Autodesk Inventor part; units mm, degrees
ref_plane "YZ Plane" through (0, 0, 0) normal (1, 0, 0) x (0, 1, 0)
ref_plane "XZ Plane" through (0, 0, 0) normal (0, 1, 0) x (-1, 0, 0)
ref_plane "XY Plane" through (0, 0, 0) normal (0, 0, 1) x (1, 0, 0)
sketch "Эскиз1" plane through (0, 0, 0) normal (0, 0, 1) x (1, 0, 0)
  line L0 (0, 0) -> (34.5, 0)
  line L1 (34.5, 0) -> (34.5, 9.5)
  line L2 (34.5, 9.5) -> (0, 9.5)
  line L3 (0, 9.5) -> (0, 0)
  line L4 (3, 9.5) -> (3, 0)
  line L5 (31.5, 9.5) -> (31.5, 0)
  line L6 (3, 3) -> (31.5, 3)
  dimension "d0" = 34.5
  dimension "d1" = 9.5
  dimension "d2" = 3
  dimension "d3" = 3
  dimension "d4" = 3
extrude "Выдавливание1" add sketch "Эскиз1" along normal blind 388 contours L3 L2 L4 L0 | L4 L6 L5 L0 | L5 L2 L1 L0
sketch "Эскиз2" plane through (0, 0, 0) normal (0, -1, 0) x (1, 0, 0)
  line L0 (0, 0) -> (34.5, 0)
  line L1 (34.5, 0) -> (34.5, 388)
  line L2 (0, 388) -> (34.5, 388)
  line L3 (0, 0) -> (0, 388)
  line L4 (17.25, 388) -> (17.25, 0)
  line L5 (22.25, 310) -> (12.25, 310)
  line L6 (12.25, 310) -> (12.25, 347)
  line L7 (12.25, 347) -> (22.25, 347)
  line L8 (22.25, 347) -> (22.25, 310)
  line L9 (22.25, 310) -> (12.25, 347) construction
  line L10 (12.25, 310) -> (22.25, 347) construction
  line L11 (12.25, 204.5) -> (22.25, 204.5)
  line L12 (22.25, 204.5) -> (22.25, 241.5)
  line L13 (22.25, 241.5) -> (12.25, 241.5)
  line L14 (12.25, 241.5) -> (12.25, 204.5)
  line L15 (12.25, 204.5) -> (22.25, 241.5) construction
  line L16 (22.25, 204.5) -> (12.25, 241.5) construction
  line L17 (22.25, 130.5) -> (12.25, 130.5)
  line L18 (12.25, 130.5) -> (12.25, 147.5)
  line L19 (12.25, 147.5) -> (22.25, 147.5)
  line L20 (22.25, 147.5) -> (22.25, 130.5)
  line L21 (22.25, 130.5) -> (12.25, 147.5) construction
  line L22 (12.25, 130.5) -> (22.25, 147.5) construction
  point P0 (17.25, 328.5)
  point P1 (17.25, 223)
  point P2 (17.25, 139)
  dimension "d8" = 10
  dimension "d9" = 37
  dimension "d10" = 41
  dimension "d11" = 10
  dimension "d12" = 37
  dimension "d13" = 68.5
  dimension "d14" = 10
  dimension "d15" = 17
  dimension "d16" = 57
extrude "Выдавливание2" cut sketch "Эскиз2" against normal blind 295 contours L17 L18 L19 L4 | L4 L19 L20 L17 | L7 L8 L5 L4 | L4 L5 L6 L7 | L11 L14 L13 L4 | L4 L13 L12 L11
fillet "Сопряжение2" radius 2 12 edges at (12.25, 1.5, 241.5) (12.25, 1.5, 204.5) (22.25, 1.5, 204.5) (22.25, 1.5, 241.5) (22.25, 1.5, 147.5) (22.25, 1.5, 130.5) (12.25, 1.5, 147.5) (12.25, 1.5, 130.5) (12.25, 1.5, 310) (12.25, 1.5, 347) (22.25, 1.5, 347) (22.25, 1.5, 310)
sketch "Эскиз3" plane through (0, 0, 388) normal (0, 0, 1) x (1, 0, 0)
  line L0 (3, 3) -> (3, 9.5)
  line L1 (3, 9.5) -> (5.5, 9.5)
  line L2 (5.5, 9.5) -> (5.5, 0)
  line L3 (5.5, 0) -> (3, 0)
  line L4 (3, 0) -> (3, 9.5)
  line L5 (31.5, 9.5) -> (31.5, 3)
  line L6 (31.5, 9.5) -> (29, 9.5)
  line L7 (29, 9.5) -> (29, 0)
  line L8 (29, 0) -> (31.5, 0)
  line L9 (31.5, 0) -> (31.5, 9.5)
  point P0 (0, 0)
  dimension "d20" = 2.5
  dimension "d21" = 2.5
extrude "Выдавливание3" add sketch "Эскиз3" against normal up to surface (388 mm away)
sketch "Эскиз4" plane through (0, 0, 0) normal (0, 0, -1) x (-1, 0, 0)
  line L0 (-34.5, 9.5) -> (-29, 9.5)
  line L1 (0, 0) -> (-34.5, 0)
  line L2 (-34.5, 9.5) -> (-32, 9.5)
  line L3 (-32, 9.5) -> (-32, 0)
  line L4 (-32, 0) -> (-34.5, 0)
  line L5 (-34.5, 0) -> (-34.5, 9.5)
  line L6 (0, 9.5) -> (0, 0)
  line L7 (0, 9.5) -> (-2.5, 9.5)
  line L8 (-2.5, 9.5) -> (-2.5, 0)
  line L9 (-2.5, 0) -> (0, 0)
  line L10 (0, 0) -> (0, 9.5)
  dimension "d24" = 2.5
  dimension "d25" = 2.5
extrude "Выдавливание4" cut sketch "Эскиз4" against normal through all
fillet "Сопряжение3" radius 2 4 edges at (5.5, 3, 194) (29, 3, 194) (29, 9.5, 194) (5.5, 9.5, 194)
sketch "Эскиз5" plane through (0, 0, 0) normal (0, 0, -1) x (-1, 0, 0)
  line L0 (52, 100) -> (-112, 100)
  line L1 (-112, 100) -> (-112, -123)
  line L2 (-112, -123) -> (52, -123)
  line L3 (52, -123) -> (52, 100)
  point P0 (0, 0)
extrude "Выдавливание5" cut sketch "Эскиз5" against normal blind 50
properties part number "2 часть направляшки 35"
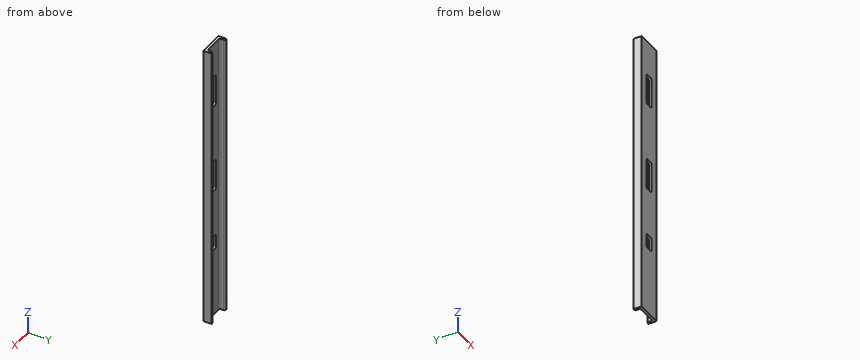
For this review, take the finished solid that the model builds, in its own axes (mm). Give positions to 0.01 mm unless a question says otherwise; leave off trailing zeros. Order: outer loops, then holes, each group sorted by start corner. A loop starts at its lowest first (then second) coordinate and runs counter-clockwise, first axis right, second up.
1) Take a section at A-A (x = 17.5). Give the boundary of the cut face in (y, z), then the cut area to 3 significant figures.
2) Wall thickness on line 1 (Z direction, x = 20.75, y = 2.25); line 2 (X direction, y = 2.75, z = 206.5); line 3 (X direction, y = 4.75, z = 366.5): over which ranges is each line inside the solid? List them lowest first.
3) Take a section at B-B (z = 331). Give the boundary of the cut face in (x, y), then the cut area to 3 significant figures.
4) Take a section at C-C (z = 89.5). Give the boundary of the cut face in (x, y).
5) Insertion check: pin 1 (5 mm diameter, centred on x = 18, z = 305.5, fed in from +Y). The pin has a flat end and moves straight along its axis. Give the tip position at first contact, or say it passes through.
Derived:
1. outline: (0, 50) - (3, 50) - (3, 130.5) - (0, 130.5) - close; (0, 147.5) - (3, 147.5) - (3, 204.5) - (0, 204.5) - close; (0, 241.5) - (3, 241.5) - (3, 310) - (0, 310) - close; (0, 347) - (3, 347) - (3, 388) - (0, 388) - close
1. area: 741 mm2
2. line 1: z = 50 to 130.56, 147.44 to 204.56, 241.44 to 310.06, 346.94 to 388
2. line 2: x = 2.5 to 12.25, 22.25 to 32
2. line 3: x = 2.5 to 5.52, 28.98 to 32
3. outline: (2.5, 0) - (12.25, 0) - (12.25, 3) - (7.5, 3) arc R2 cw to (5.5, 5) - (5.5, 7.5) arc R2 ccw to (3.5, 9.5) - (2.5, 9.5) - close; (22.25, 0) - (32, 0) - (32, 9.5) - (31, 9.5) arc R2 ccw to (29, 7.5) - (29, 5) arc R2 cw to (27, 3) - (22.25, 3) - close
3. area: 97.5 mm2
4. outline: (2.5, 0) - (32, 0) - (32, 9.5) - (31, 9.5) arc R2 ccw to (29, 7.5) - (29, 5) arc R2 cw to (27, 3) - (7.5, 3) arc R2 cw to (5.5, 5) - (5.5, 7.5) arc R2 ccw to (3.5, 9.5) - (2.5, 9.5) - close
5. pin 1: stops at y = 3
